Input: part model. Units: mm. Frame: model coordinates. Face numbers are marked on the shaded views. Round coordinates to 2 decimals unless told otherwise and drop trailing zeros. Loops run counter-clockwise (first coordinate to the right, second up) from the corner with the lowest first, then second, coordinate; pieces in that order, holes last. Notation, with made-up numbers: (47.5, -22.75) -> (59.5, -22.75) arc R25 cw to (59.5, -3.75) -> close; hole circle Ø11 at (57, -39). An arc over 180 degrees is marked (long way). Answer as a JSON object with one key per item and string values. Group by question number.
Item 1: Draft query along X for the marked faces 1, 2, 3 and 4. Return one class per face: released by +X, released by -X, zero draft, split by the parting line, or undercut.
Item 2: Section query D-D on x = -13. Return loops of the section in (y, z) (3 decimals).
Item 3: Section query B-B on y = -23. Return loops of the section in (x, z) (3 decimals).
Item 4: Section query A-A on x = 35.5. Return loops of the section in (y, z) (3 decimals).
Item 5: Material intervals for line 1 (Y direction, x = -19, z = 1.75) (3 decimals); line 2 (Y direction, x = -20, z = 2.5) (3 decimals); line 3 (Z direction, x = -53.5, y = 2), sorted ascending. Write a range as [from, to].
Item 6: Section query C-C on y = 0.5. Return loops of the section in (x, z) (1 decimal).
Item 7: Pin query (flat end, axial travel): pin 1 (3 mm diameter, centred on y = 28, z = 1, fed in from -X); pin 2 (4 mm diameter, centred on x = -2.5, z = 21, fed in from +Y); pin 3 (2 mm diameter, centred on x = 32.5, z = 0.5, fed in from -Y); pin 4 (12 mm diameter, centred on x = 35.5, y = 38.5, fed in from +Z). Return the tip coordinate at first contact, or that it passes through.
from build123d import *

# Parameters (mm, degrees)
F1_DEPTH      = 27.94
F2_W          = 59.69
F2_H          = 6.35
F2_W_2        = 6.35
F3_DEPTH      = 2.54
F4_W          = 5.08
F4_H          = 20.32
F5_DEPTH      = 62.866
F5_DEPTH_BACK = 62.866
F6_T1_DEPTH   = 20.32
F8_DEPTH      = 3.5254948624
F8_DEPTH_BACK = 3.5254948624


# Not quite as in the source:
# - a fillet or chamfer that OpenCascade refuses, or shapes differently, is made with other operations: its cross-section is extruded or revolved along the edge and cut away or added


with BuildPart() as f1:
    # F0 (on Top) → F1 (new body)
    with BuildSketch(Plane.XY):
        with BuildLine():
            Line((-70.9619581652, -6.2947835132), (-60.8714999798, -15.7056905359))
            ThreePointArc((-60.8714999798, -15.7056905359), (-62.3646336926, -7.9158505156), (-62.865, 0))
            Line((-62.865, 0), (-62.865, -3.175))
            Line((-62.865, -3.175), (-70.254501201, -4.1059896424))
            ThreePointArc((-70.254501201, -4.1059896424), (-71.304196006, -4.9754379298), (-70.9619581652, -6.2947835132))
        make_face()
        with BuildLine():
            ThreePointArc((-58.2446298794, 15.7056905359), (0, 60.325), (58.2446298794, 15.7056905359))
            Line((58.2446298794, 15.7056905359), (60.8714999798, 15.7056905359))
            ThreePointArc((60.8714999798, 15.7056905359), (0, 62.865), (-60.8714999798, 15.7056905359))
            Line((-60.8714999798, 15.7056905359), (-58.2446298794, 15.7056905359))
        make_face()
        with BuildLine():
            ThreePointArc((-58.2446298794, -15.7056905359), (-60.325, 0), (-58.2446298794, 15.7056905359))
            Line((-58.2446298794, 15.7056905359), (-60.8714999798, 15.7056905359))
            ThreePointArc((-60.8714999798, 15.7056905359), (-62.3646336926, 7.9158505156), (-62.865, 0))
            ThreePointArc((-62.865, 0), (-62.3646336926, -7.9158505156), (-60.8714999798, -15.7056905359))
            Line((-60.8714999798, -15.7056905359), (-58.2446298794, -15.7056905359))
        make_face()
        with BuildLine():
            Line((60.8714999798, -15.7056905359), (58.2446298794, -15.7056905359))
            ThreePointArc((58.2446298794, -15.7056905359), (0, -60.325), (-58.2446298794, -15.7056905359))
            Line((-58.2446298794, -15.7056905359), (-60.8714999798, -15.7056905359))
            ThreePointArc((-60.8714999798, -15.7056905359), (0, -62.865), (60.8714999798, -15.7056905359))
        make_face()
        with BuildLine():
            ThreePointArc((58.2446298794, 15.7056905359), (59.8026459384, 7.9214369758), (60.325, 0))
            ThreePointArc((60.325, 0), (59.8026459384, -7.9214369758), (58.2446298794, -15.7056905359))
            Line((58.2446298794, -15.7056905359), (60.8714999798, -15.7056905359))
            ThreePointArc((60.8714999798, -15.7056905359), (62.3646336926, -7.9158505156), (62.865, 0))
            ThreePointArc((62.865, 0), (62.3646336926, 7.9158505156), (60.8714999798, 15.7056905359))
            Line((60.8714999798, 15.7056905359), (58.2446298794, 15.7056905359))
        make_face()
        with BuildLine():
            Line((70.9619581652, 6.2947835132), (60.8714999798, 15.7056905359))
            ThreePointArc((60.8714999798, 15.7056905359), (62.3646336926, 7.9158505156), (62.865, 0))
            Line((62.865, 0), (62.865, 3.175))
            Line((62.865, 3.175), (70.254501201, 4.1059896424))
            ThreePointArc((70.254501201, 4.1059896424), (71.304196006, 4.9754379298), (70.9619581652, 6.2947835132))
        make_face()
        with BuildLine():
            ThreePointArc((62.865, 0), (62.3646336926, -7.9158505156), (60.8714999798, -15.7056905359))
            Line((60.8714999798, -15.7056905359), (70.9619581652, -6.2947835132))
            ThreePointArc((70.9619581652, -6.2947835132), (71.304196006, -4.9754379298), (70.254501201, -4.1059896424))
            Line((70.254501201, -4.1059896424), (62.865, -3.175))
            Line((62.865, -3.175), (62.865, 0))
        make_face()
        with BuildLine():
            ThreePointArc((-62.865, 0), (-62.3646336926, 7.9158505156), (-60.8714999798, 15.7056905359))
            Line((-60.8714999798, 15.7056905359), (-70.9619581652, 6.2947835132))
            ThreePointArc((-70.9619581652, 6.2947835132), (-71.304196006, 4.9754379298), (-70.254501201, 4.1059896424))
            Line((-70.254501201, 4.1059896424), (-62.865, 3.175))
            Line((-62.865, 3.175), (-62.865, 0))
        make_face()
        with BuildLine():
            ThreePointArc((58.2446298794, -15.7056905359), (59.8026459384, -7.9214369758), (60.325, 0))
            ThreePointArc((60.325, 0), (59.8026459384, 7.9214369758), (58.2446298794, 15.7056905359))
            Line((58.2446298794, 15.7056905359), (58.2446298794, -15.7056905359))
        make_face()
        with BuildLine():
            Line((-58.2446298794, -15.7056905359), (-58.2446298794, 15.7056905359))
            ThreePointArc((-58.2446298794, 15.7056905359), (-60.325, 0), (-58.2446298794, -15.7056905359))
        make_face()
    extrude(amount=F1_DEPTH)

    # F2 (on face) → F3 (join)
    with BuildSketch(Plane(origin=(0, 0, 0), x_dir=(1, 0, 0), z_dir=(0, 0, -1))):
        with Locations((33.02, 0)):
            Rectangle(F2_W, F2_H)
        Rectangle(F2_W_2, F2_H)
        with Locations((-33.02, 0)):
            Rectangle(F2_W, F2_H)
        with BuildLine():
            Line((-3.175, 3.175), (3.175, 3.175))
            Line((3.175, 3.175), (3.175, 60.2413894262))
            ThreePointArc((3.175, 60.2413894262), (0, 60.325), (-3.175, 60.2413894262))
            Line((-3.175, 60.2413894262), (-3.175, 3.175))
        make_face()
        with BuildLine():
            Line((3.175, -60.2413894262), (3.175, -3.175))
            Line((3.175, -3.175), (-3.175, -3.175))
            Line((-3.175, -3.175), (-3.175, -60.2413894262))
            ThreePointArc((-3.175, -60.2413894262), (0, -60.325), (3.175, -60.2413894262))
        make_face()
    extrude(amount=-F3_DEPTH)

    # F4 (on Front) → F5 (cut, two sides)
    with BuildSketch(Plane.XZ) as f5_sk:
        with Locations((-12.7, 13.97)):
            Rectangle(F4_W, F4_H)
        with Locations((12.7, 13.97)):
            Rectangle(F4_W, F4_H)
    extrude(amount=-F5_DEPTH, mode=Mode.SUBTRACT)
    extrude(f5_sk.sketch, amount=F5_DEPTH_BACK, mode=Mode.SUBTRACT)

    # F6: fillet of radius 2.54 on 8 edges, made by hand

    # F6_s2 → F6_t1 (cut)
    with BuildSketch(Plane.XY.offset(3.81)):
        with BuildLine():
            ThreePointArc((18.4281257881, 60.1033477016), (16.4693425511, 59.9059132544), (15.24, 58.3682107401))
            Line((15.24, 58.3682107401), (15.24, 60.9897583615))
            ThreePointArc((15.24, 60.9897583615), (16.8398962136, 60.5675335515), (18.4281257881, 60.1033477016))
        make_face()
        with BuildLine():
            ThreePointArc((-18.4281257881, 60.1033477016), (-16.4693425511, 59.9059132544), (-15.24, 58.3682107401))
            Line((-15.24, 58.3682107401), (-15.24, 60.9897583615))
            ThreePointArc((-15.24, 60.9897583615), (-16.8398962136, 60.5675335515), (-18.4281257881, 60.1033477016))
        make_face()
        with BuildLine():
            ThreePointArc((7.3366965941, 59.8771952256), (9.1895995283, 60.3814871069), (10.16, 62.038557567))
            Line((10.16, 62.038557567), (10.16, 59.4632661817))
            ThreePointArc((10.16, 59.4632661817), (8.7507960918, 59.6869264811), (7.3366965941, 59.8771952256))
        make_face()
        with BuildLine():
            ThreePointArc((-7.3366965941, 59.8771952256), (-9.1895995283, 60.3814871069), (-10.16, 62.038557567))
            Line((-10.16, 62.038557567), (-10.16, 59.4632661817))
            ThreePointArc((-10.16, 59.4632661817), (-8.7507960918, 59.6869264811), (-7.3366965941, 59.8771952256))
        make_face()
        with BuildLine():
            ThreePointArc((-18.4281257881, -60.1033477016), (-16.4693425511, -59.9059132544), (-15.24, -58.3682107401))
            Line((-15.24, -58.3682107401), (-15.24, -60.9897583615))
            ThreePointArc((-15.24, -60.9897583615), (-16.8398962136, -60.5675335515), (-18.4281257881, -60.1033477016))
        make_face()
        with BuildLine():
            ThreePointArc((18.4281257881, -60.1033477016), (16.4693425511, -59.9059132544), (15.24, -58.3682107401))
            Line((15.24, -58.3682107401), (15.24, -60.9897583615))
            ThreePointArc((15.24, -60.9897583615), (16.8398962136, -60.5675335515), (18.4281257881, -60.1033477016))
        make_face()
        with BuildLine():
            ThreePointArc((7.3366965941, -59.8771952256), (9.1895995283, -60.3814871069), (10.16, -62.038557567))
            Line((10.16, -62.038557567), (10.16, -59.4632661817))
            ThreePointArc((10.16, -59.4632661817), (8.7507960918, -59.6869264811), (7.3366965941, -59.8771952256))
        make_face()
        with BuildLine():
            ThreePointArc((-7.3366965941, -59.8771952256), (-9.1895995283, -60.3814871069), (-10.16, -62.038557567))
            Line((-10.16, -62.038557567), (-10.16, -59.4632661817))
            ThreePointArc((-10.16, -59.4632661817), (-8.7507960918, -59.6869264811), (-7.3366965941, -59.8771952256))
        make_face()
    extrude(amount=F6_T1_DEPTH, mode=Mode.SUBTRACT)

    # F7 (on Front) → F8 (join, two sides)
    with BuildSketch(Plane.XZ) as f8_sk:
        with BuildLine():
            ThreePointArc((65.0278285183, 17.4625), (65.4371804989, 23.0089829265), (62.865, 27.94))
            Line((62.865, 27.94), (62.865, 0))
            ThreePointArc((62.865, 0), (65.4371804989, 4.9310170735), (65.0278285183, 10.4775))
            ThreePointArc((65.0278285183, 10.4775), (64.4086903111, 13.97), (65.0278285183, 17.4625))
        make_face()
        with BuildLine():
            ThreePointArc((-65.0278285183, 10.4775), (-65.4371804989, 4.9310170735), (-62.865, 0))
            Line((-62.865, 0), (-62.865, 27.94))
            ThreePointArc((-62.865, 27.94), (-65.4371804989, 23.0089829265), (-65.0278285183, 17.4625))
            ThreePointArc((-65.0278285183, 17.4625), (-64.4086903111, 13.97), (-65.0278285183, 10.4775))
        make_face()
    extrude(amount=F8_DEPTH)
    extrude(f8_sk.sketch, amount=-F8_DEPTH_BACK)


solid = f1.part
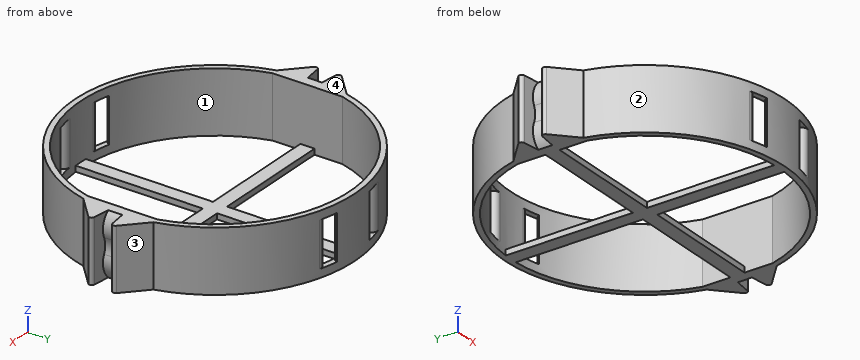
Solved:
{
 "1": {"face 1": "undercut", "face 2": "split by the parting line", "face 3": "released by +X", "face 4": "zero draft"},
 "2": {"outline": "(-61.506, 0) -> (-58.908, 0) -> (-58.908, 3.81) -> (-61.506, 3.81) -> close; (-61.506, 24.13) -> (-58.908, 24.13) -> (-58.908, 27.94) -> (-61.506, 27.94) -> close; (-3.175, 0) -> (3.175, 0) -> (3.175, 2.54) -> (-3.175, 2.54) -> close; (58.908, 0) -> (61.506, 0) -> (61.506, 3.81) -> (58.908, 3.81) -> close; (58.908, 24.13) -> (61.506, 24.13) -> (61.506, 27.94) -> (58.908, 27.94) -> close"},
 "3": {"outline": "(-58.506, 0) -> (-55.768, 0) -> (-55.768, 27.94) -> (-58.506, 27.94) -> close; (-3.175, 0) -> (3.175, 0) -> (3.175, 2.54) -> (-3.175, 2.54) -> close; (55.768, 0) -> (58.506, 0) -> (58.506, 27.94) -> (55.768, 27.94) -> close"},
 "4": {"outline": "(-51.882, 0) -> (-48.774, 0) -> (-48.774, 27.94) -> (-51.882, 27.94) -> close; (-3.175, 0) -> (3.175, 0) -> (3.175, 2.54) -> (-3.175, 2.54) -> close; (48.774, 0) -> (51.882, 0) -> (51.882, 27.94) -> (48.774, 27.94) -> close"},
 "5": {"line 1": "[-59.925, -57.255], [-3.175, 3.175], [57.255, 59.925]", "line 2": "[-59.599, -56.913], [-3.175, 3.175], [56.913, 59.599]", "line 3": "[0, 2.54]"},
 "6": {"outline": "(-65, 10.5) arc R10.2 ccw to (-62.9, 0) -> (62.9, 0) arc R10.2 ccw to (65, 10.5) arc R10.2 cw to (65, 17.5) arc R10.2 ccw to (62.9, 27.9) -> (58.2, 27.9) -> (58.2, 2.5) -> (-58.2, 2.5) -> (-58.2, 27.9) -> (-62.9, 27.9) arc R10.2 ccw to (-65, 17.5) arc R10.2 cw to start"},
 "7": {"pin 1": "x = -57.01", "pin 2": "y = 62.86", "pin 3": "y = -54.4", "pin 4": "through"}
}
